Read the model definition and answer for the solid it produces. Units are mm, in the model's axes. A direction names the side the tool comes from. Coordinates: 2 decimals unless noted, no trailing zeros. Order: outer loops, then holes, each group sorted by start corner. A loop starts at its lowest first (then second) coordinate and runs counter-clockwise, first axis right, second up. Notation, with made-up numbers: (36, -6) -> (66, -6) arc R26 cw to (66, 30) -> close; hole circle Ø1 at (4, 13.25). An arc over 180 degrees is marked (long way). Answer in a Markdown table with one row per item.
from build123d import *

# Parameters (mm, degrees)
SKETCH_1_R          = 1.5
EXTRUDE_1_DEPTH     = 3
CHAMFER_1_SIZE      = 7
FILLET_1_R          = 5
SKETCH_3_W          = 60
SKETCH_3_H          = 60
SKETCH_3_R          = 1.5
SKETCH_3_R_2        = 20
SKETCH_3_W_2        = 80
SKETCH_3_H_2        = 12
CUT_EXTRUDE_1_DEPTH = 3
FILLET_3_R          = 10
CHAMFER_2_SIZE      = 12
SKETCH_4_R          = 1.5
CUT_EXTRUDE_2_DEPTH = 10


with BuildPart() as part:
    # 草图1 → 凸台-拉伸1 (new body)
    with BuildSketch(Plane(origin=(0, 0, 0), x_dir=(1, 0, 0), z_dir=(0, 1, 0))):
        Polygon((-62.5, 62.5), (-62.5, -62.5), (62.5, -62.5), (62.5, 62.5), (43, 62.5), (43, 125), (-43, 125), (-43, 62.5), align=None)
        with Locations(Location((-56.5, -50.843145751, 0), (0, 0, 270))):
            Circle(SKETCH_1_R, mode=Mode.SUBTRACT)
        with Locations(Location((-50.843145751, -56.5, 0), (0, 0, 270))):
            Circle(SKETCH_1_R, mode=Mode.SUBTRACT)
        with Locations(Location((50.843145751, -56.5, 0), (0, 0, 270))):
            Circle(SKETCH_1_R, mode=Mode.SUBTRACT)
        with Locations(Location((56.5, -50.843145751, 0), (0, 0, 270))):
            Circle(SKETCH_1_R, mode=Mode.SUBTRACT)
        with Locations(Location((-56.5, 50.843145751, 0), (0, 0, 270))):
            Circle(SKETCH_1_R, mode=Mode.SUBTRACT)
        with Locations(Location((-50.843145751, 56.5, 0), (0, 0, 270))):
            Circle(SKETCH_1_R, mode=Mode.SUBTRACT)
        with Locations(Location((56.5, 50.843145751, 0), (0, 0, 270))):
            Circle(SKETCH_1_R, mode=Mode.SUBTRACT)
        with Locations(Location((50.843145751, 56.5, 0), (0, 0, 270))):
            Circle(SKETCH_1_R, mode=Mode.SUBTRACT)
        with Locations(Location((38, 117, 0), (0, 0, 270))):
            Circle(SKETCH_1_R, mode=Mode.SUBTRACT)
        with Locations(Location((-38, 117, 0), (0, 0, 270))):
            Circle(SKETCH_1_R, mode=Mode.SUBTRACT)
    extrude(amount=EXTRUDE_1_DEPTH)

    # 倒角1
    chamfer_1_edges = [part.edges().sort_by_distance(p)[0] for p in [
        (-62.5, 1.5, 62.5),
        (-62.5, 1.5, -62.5),
        (62.5, 1.5, -62.5),
        (62.5, 1.5, 62.5),
    ]]
    chamfer(chamfer_1_edges, length=CHAMFER_1_SIZE)

    # 圆角1
    fillet_1_edges = [part.edges().sort_by_distance(p)[0] for p in [
        (-43, 1.5, -62.5),
        (-43, 1.5, -125),
        (43, 1.5, -125),
        (43, 1.5, -62.5),
    ]]
    fillet(fillet_1_edges, radius=FILLET_1_R)

    # 草图3 → 切除-拉伸1 (cut)
    with BuildSketch(Plane(origin=(0, 3, 0), x_dir=(1, 0, 0), z_dir=(0, 1, 0))):
        Rectangle(SKETCH_3_W, SKETCH_3_H)
        with Locations(Location((-45.5, 45.5, 0), (0, 0, 270))):
            Circle(SKETCH_3_R)
        with Locations(Location((45.5, 45.5, 0), (0, 0, 270))):
            Circle(SKETCH_3_R)
        with Locations(Location((45.5, -45.5, 0), (0, 0, 270))):
            Circle(SKETCH_3_R)
        with Locations(Location((-45.5, -45.5, 0), (0, 0, 270))):
            Circle(SKETCH_3_R)
        with Locations(Location((0, 90, 0), (0, 0, 270))):
            Circle(SKETCH_3_R_2)
        with Locations((0, -56.5)):
            Rectangle(SKETCH_3_W_2, SKETCH_3_H_2)
    extrude(amount=-CUT_EXTRUDE_1_DEPTH, mode=Mode.SUBTRACT)

    # 圆角3
    fillet_3_edges = [part.edges().sort_by_distance(p)[0] for p in [
        (30, 1.5, 30),
        (-30, 1.5, 30),
        (-30, 1.5, -30),
        (30, 1.5, -30),
    ]]
    fillet(fillet_3_edges, radius=FILLET_3_R)

    # 倒角2
    chamfer_2_edges = [part.edges().sort_by_distance(p)[0] for p in [
        (40, 1.5, 50.5),
        (-40, 1.5, 50.5),
    ]]
    chamfer(chamfer_2_edges, length=CHAMFER_2_SIZE - 0.0001)  # a hair under: the kernel refuses the full size

    # 草图4 → 切除-拉伸2 (cut)
    with BuildSketch(Plane(origin=(0, 3, 0), x_dir=(1, 0, 0), z_dir=(0, 1, 0))):
        with Locations(Location((-41, 32.5, 0), (0, 0, 270))):
            Circle(SKETCH_4_R)
        with Locations(Location((44, 30, 0), (0, 0, 270))):
            Circle(SKETCH_4_R)
        with Locations(Location((-39, -27, 0), (0, 0, 270))):
            Circle(SKETCH_4_R)
        with Locations(Location((39, -27, 0), (0, 0, 270))):
            Circle(SKETCH_4_R)
    extrude(amount=-CUT_EXTRUDE_2_DEPTH, mode=Mode.SUBTRACT)


solid = part.part
Q1. The part is cut by section C-C (x = -17.5). Write down the section's boundary in (y, z), then the cut area to 3 significant figures.
Outcome:
| item | result |
|---|---|
| outline | (0, -125) -> (3, -125) -> (3, -99.68) -> (0, -99.68) -> close; (0, -80.32) -> (3, -80.32) -> (3, -30) -> (0, -30) -> close; (0, 30) -> (3, 30) -> (3, 50.5) -> (0, 50.5) -> close |
| area | 288 mm² |
Q2. Consider line 1 (Z direction, x = -1, y = 1.4); line 2 (X direction, y = 1.5, z = 45.5); line 3 (X direction, y = 2.1, z = -117). Determine where each line is inside the solid, lowest interval first.
Outcome:
| item | result |
|---|---|
| line 1 | -125 to -109.97, -70.03 to -30, 30 to 50.5 |
| line 2 | -62.5 to -47, -44 to 44, 47 to 62.5 |
| line 3 | -43 to -39.5, -36.5 to 36.5, 39.5 to 43 |
Q3. For a pull along Z with two mould halves and no side action, classify faces 4 (the face through (-59, 1, 59)), 5 (the face through (-26.99, 1.48, -27.15)), 6 (the face through (-42, 2, -123)), 7 (the face through (-1, 3, -33)) as pulls with the +Z half, pulls with the -Z half, needs draft (parallel to the pull), parting line crosses it, or undercut.
Outcome:
| item | result |
|---|---|
| face 4 | pulls with the +Z half |
| face 5 | undercut |
| face 6 | pulls with the -Z half |
| face 7 | needs draft |
Q4. For faces 1 (the face through (-26.99, 1.48, 27.15)), 2 (the face through (59, 1, -59)), 3 (the face through (-34.1, 1.5, 56.6)), determine the directions among +Z, -Z, +X, -X, +Y, -Y from which every point of the face is accessible in a straight line to the end or side of a thin tool.
Outcome:
| item | result |
|---|---|
| face 1 | +Y, -Y |
| face 2 | -Z, +X, +Y, -Y |
| face 3 | +Z, +Y, -Y |
Q5. The part is cut by section D-D (y = 2.5). Give the number of separate pieces and of enclosed holes in the cut face, then the cut area to 3 significant figures.
Outcome:
| item | result |
|---|---|
| separate pieces | 1 |
| enclosed holes | 20 |
| area | 15,200 mm² |
Q6. The part is cut by section A-A (x = 0). Write down the section's boundary in (y, z), then the cut area to 4 significant figures.
Outcome:
| item | result |
|---|---|
| outline | (0, -125) -> (3, -125) -> (3, -110) -> (0, -110) -> close; (0, -70) -> (3, -70) -> (3, -30) -> (0, -30) -> close; (0, 30) -> (3, 30) -> (3, 50.5) -> (0, 50.5) -> close |
| area | 226.5 mm² |
Q7. The part is cut by section B-B (z = -84). Write down the section's boundary in (x, y).
Outcome:
| item | result |
|---|---|
| outline | (-43, 0) -> (-19.08, 0) -> (-19.08, 3) -> (-43, 3) -> close; (19.08, 0) -> (43, 0) -> (43, 3) -> (19.08, 3) -> close |
